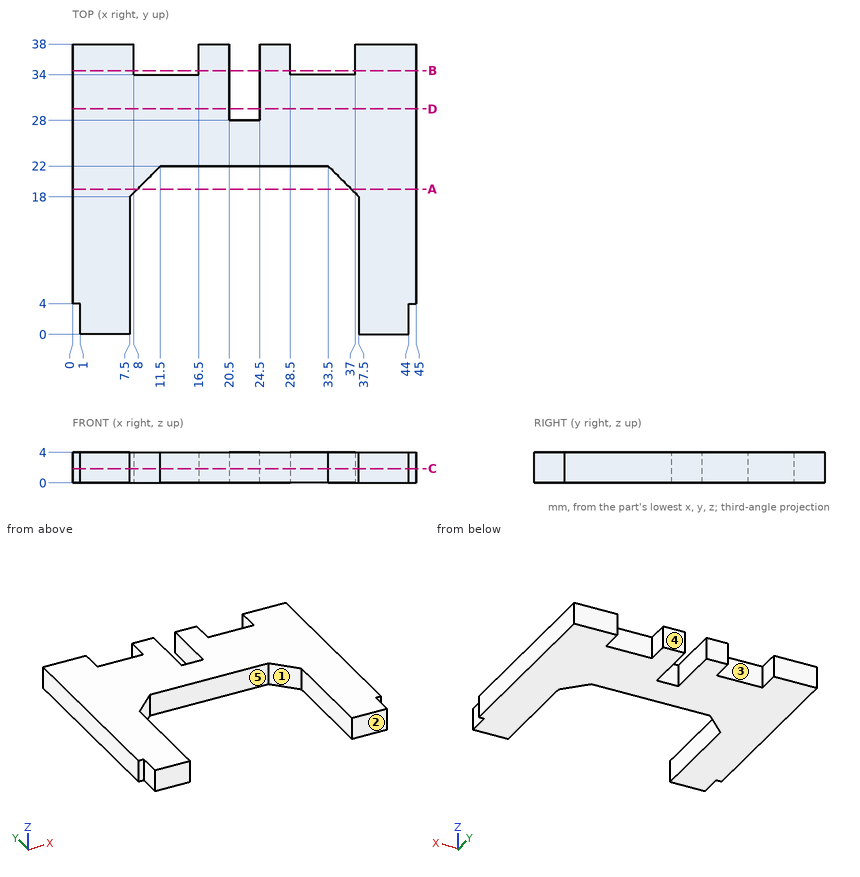
Print and shaded views of the part. All mm, measured from the part's lowest x, y and z. A direction names the side the tool comes from. Give positions to 0.01 mm unless a question says otherwise; leave off trailing zeros. Loops run counter-clockwise (first coordinate to the right, second up) from the corner with the lowest first, then second, coordinate; pieces in that order, holes last. Notation, with made-up numbers: (45, 44.25) - (86, 44.25) arc R21 ccw to (86, 68.25) - close; hole circle Ø3 at (-20, 76.5). An arc over 180 degrees is marked (long way). Use a Markdown table: item, result.
(1) Which spindle directions (+Z, -Z, +X, -X, +Y, -Y) get a long thin tool onto all of the face, cutting with end or side? Do the marked faces 3, 4 and 5. Say none if no direction does.
Taken from the geometry:
| item | result |
|---|---|
| face 3 | +Z, -Z, +Y |
| face 4 | +Z, -Z, +X, -X, +Y |
| face 5 | +Z, -Z, -Y |
(2) Band-saw the part on A-A (y = 19). Give the cut face in (x, z).
Taken from the geometry:
| item | result |
|---|---|
| outline | (0, 0) - (8.5, 0) - (8.5, 4) - (0, 4) - close; (36.5, 0) - (45, 0) - (45, 4) - (36.5, 4) - close |
(3) Drop flat-ended pins along their axis: pin 1 Ø2 at (y, z) = (2, 2.5) entering from -X; pin 2 Ø2 at (x, z) = (22.5, 3) entering from +Y; pin 3 Ø1 at (x, z) = (23, 0.5) entering from -Y. Give the stop position or say it passes through.
Taken from the geometry:
| item | result |
|---|---|
| pin 1 | x = 1 |
| pin 2 | y = 28 |
| pin 3 | y = 22 |
(4) Band-saw the part on B-B (y = 34.5). Give the cut face in (x, z), and give its area (3 significant figures).
Taken from the geometry:
| item | result |
|---|---|
| outline | (0, 0) - (8, 0) - (8, 4) - (0, 4) - close; (16.5, 0) - (20.5, 0) - (20.5, 4) - (16.5, 4) - close; (24.5, 0) - (28.5, 0) - (28.5, 4) - (24.5, 4) - close; (37, 0) - (45, 0) - (45, 4) - (37, 4) - close |
| area | 96.0 mm2 |
(5) Band-saw the part on D-D (y = 29.5). Give the cut face in (x, z), and give its area (3 significant figures).
Taken from the geometry:
| item | result |
|---|---|
| outline | (0, 0) - (20.5, 0) - (20.5, 4) - (0, 4) - close; (24.5, 0) - (45, 0) - (45, 4) - (24.5, 4) - close |
| area | 164 mm2 |
(6) Pull direction X, two halves, no side cores. Call the marked faces 1 and 2: +X half, -X half, draft (parallel to the pull), parting line (faces both ways), or undercut.
Taken from the geometry:
| item | result |
|---|---|
| face 1 | undercut |
| face 2 | draft |
(7) Band-saw the part on C-C (z = 1.85). Give the cut face in (x, y), and give its area (3 significant figures).
Taken from the geometry:
| item | result |
|---|---|
| outline | (0, 4) - (1, 4) - (1, 0) - (7.5, 0) - (7.5, 18) - (11.5, 22) - (33.5, 22) - (37.5, 18) - (37.5, 0) - (44, 0) - (44, 4) - (45, 4) - (45, 38) - (37, 38) - (37, 34) - (28.5, 34) - (28.5, 38) - (24.5, 38) - (24.5, 28) - (20.5, 28) - (20.5, 38) - (16.5, 38) - (16.5, 34) - (8, 34) - (8, 38) - (0, 38) - close |
| area | 950 mm2 |
(8) Wall check: line 1 along X through (y, z) = (34.5, 1.05); line 2 along X through (y, z) = (17.5, 2.2); line 3 along X through (y, z) = (33, 0.3). Give the ranges that are in metal, low to high.
Taken from the geometry:
| item | result |
|---|---|
| line 1 | 0 to 8, 16.5 to 20.5, 24.5 to 28.5, 37 to 45 |
| line 2 | 0 to 7.5, 37.5 to 45 |
| line 3 | 0 to 20.5, 24.5 to 45 |
